Source: CAD feature listing. Evaluate the final solid. Frame: model axes, mm. A direction names the side the tool comes from. Give positions to 0.01 mm unless a question says otherwise; leave off trailing zeros. Write each loop counter-clockwise with the first axis right and the second up, starting at its lowest first coordinate (ties: lowest second). Pieces come first, ordered by that corner, then holes. Notation, with made-up numbers: M 79.5,17.5 L 132.5,17.5 A18 ccw 132.5,50.5 Z; hole C 89,-23 d3. An arc over 180 degrees is marked long. Answer as a JSON object with one key per item and string values. Group by question number.
Autodesk Inventor part; units mm, degrees
ref_plane "shaft_to_bearing_XY" through (0, 0, 0) normal (1, 0, 0) x (0, 0, -1)
ref_plane "shaft_to_bearing_YZ" through (0, 0, 0) normal (0, 0, -1) x (0, 1, 0)
ref_plane "shaft_to_bearing_ZX" through (0, 0, 0) normal (0, 1, 0) x (1, 0, 0)
sketch "Sketch_1" plane through (0, 0, 0) normal (0, 0, 1) x (1, 0, 0)
  line L0 (1, 0) -> (-4.8, 0)
  line L1 (-4.8, 0) -> (-4.8, 1.8)
  line L2 (-4.8, 1.8) -> (-4.6, 2)
  line L3 (-4.6, 2) -> (-0.2, 2)
  arc A0 (-0.2, 2) -> (0, 2.2) centre (-0.2, 2.2) ccw
  line L4 (0, 2.2) -> (0, 2.8)
  line L5 (0, 2.8) -> (1, 2.8)
  line L6 (1, 2.8) -> (1, 0)
  line L7 (1, 0) -> (-4.8, 0)
revolve "Revolution1" add sketch "Sketch_1" angle 360 about axis through (1, 0, 0) along (1, 0, 0)
sketch "Sketch_5" plane through (0, 0, 0) normal (0, 0, 1) x (1, 0, 0)
  line L0 (9, 0) -> (1, 0)
  line L1 (1, 0) -> (1, 2)
  line L2 (1, 2) -> (8.5705, 2)
  line L3 (8.5705, 2) -> (9, 1.5705)
  line L4 (9, 1.5705) -> (9, 0)
  line L5 (9, 0) -> (1, 0)
revolve "Revolution2" add sketch "Sketch_5" angle 360 about axis through (9, 0, 0) along (1, 0, 0)
thread "Thread1"
sketch "Sketch_2" plane through (-4.8, 0, 0) normal (1, 0, 0) x (0, 0, -1)
  line L0 (-1, -0.5774) -> (0, -1.1547)
  line L1 (0, -1.1547) -> (1, -0.5774)
  line L2 (1, -0.5774) -> (1, 0.5774)
  line L3 (1, 0.5774) -> (0, 1.1547)
  line L4 (0, 1.1547) -> (-1, 0.5774)
  line L5 (-1, 0.5774) -> (-1, -0.5774)
extrude "Extrusion1" cut sketch "Sketch_2" along normal blind 1.5
sketch "Sketch_3" plane through (0, 0, 0) normal (0, 0, 1) x (1, 0, 0)
  line L0 (-2.7226, 0) -> (-3.3, 0)
  line L1 (-3.3, 0) -> (-3.3, 1)
  line L2 (-3.3, 1) -> (-2.7226, 0)
  line L3 (-2.7226, 0) -> (-3.3, 0)
revolve "Revolution3" cut sketch "Sketch_3" angle 360 about axis through (-2.7226, 0, 0) along (1, 0, 0)
ref_plane "shaft_to_bearing_XY" through (0, 0, 0) normal (1, 0, 0) x (0, 0, -1)
ref_plane "shaft_to_bearing_YZ" through (0, 0, 0) normal (0, 0, -1) x (0, 1, 0)
ref_plane "shaft_to_bearing_ZX" through (0, 0, 0) normal (0, 1, 0) x (1, 0, 0)
properties part number "E-NTBGT13-8_b"
(1) Contact query for flat-ended pins moving along their axis: pin 1 Ø3 at (x, y) = (6, 1.5) entering from -Z; pin 2 Ø0.6 at (y, z) = (-0.5, 0) entering from -X; pin 3 Ø1 at (x, z) = (5, 0.5) entering from -Y. Output: stop coordinate, or through.
(2) Section A-A, the plane x = -3.5. Return loops of the section in (y, z).
(3) Ray query, L1, parallel to X at y = 0.7, z = 2.1; L2, parallel to Z at x = 1.5, y = 0; L3, parallel to X at y = -0.1, z = 0.9. Return the intervals inside material, ascending. Write a range as [from, to].
(4) Pull-direction query (Z, two-part tool) for faces 4 (the cylindrical face through (5, 0, -2)), 5 (the flat face through (9, 0, 0)), 6 (the flat face through (-4, 0, 1)), 7 (the flat face through (-4.06, -0.87, -0.49)); classes: pulls with the +Z half, pulls with the -Z half, needs draft (parallel to the pull), parting line crosses it, or undercut.
(5) Section C-C, the plane z = -2.35. Return loops of the section in (x, y), plus the area to 3 significant figures.
(6) Section B-B, the plane x = 5.5. Return loops of the section in (y, z), plus the area to 3 significant figures.
(7) Access query for faces 1 (the flat face through (-4.8, 1, -1)), 2 (the flat face through (-4.06, 0.86, -0.51)), 3 (the flat face through (1, -2, 1)). Directions: +Z, -Z, +X, -X, +Y, -Y. A direction counts if a zero-diameter tool reaches every point of the face in a straight line with its end or side. Return the directions, or none.
Reported:
{
 "1": {"pin 1": "stops at z = -2", "pin 2": "stops at x = -3.18", "pin 3": "stops at y = -2"},
 "2": {"outline": "C 0,0 d4; hole M -1.15,0 L -0.58,-1 L 0.58,-1 L 1.15,0 L 0.58,1 L -0.58,1 Z"},
 "3": {"L1": "x = [0, 1]", "L2": "z = [-2, 2]", "L3": "x = [-3.25, 9]"},
 "4": {"face 4": "parting line crosses it", "face 5": "needs draft", "face 6": "undercut", "face 7": "undercut"},
 "5": {"outline": "M 0,-1.52 L 1,-1.52 L 1,1.52 L 0,1.52 Z", "area": "3.04 mm2"},
 "6": {"outline": "C 0,0 d4", "area": "12.6 mm2"},
 "7": {"face 1": "+Z, -Z, -X, +Y, -Y", "face 2": "-X", "face 3": "+X"}
}
